Autodesk Inventor part; units mm, degrees
ref_plane "YZ Plane" through (0, 0, 0) normal (1, 0, 0) x (0, 1, 0)
ref_plane "XZ Plane" through (0, 0, 0) normal (0, 1, 0) x (-1, 0, 0)
ref_plane "XY Plane" through (0, 0, 0) normal (0, 0, 1) x (1, 0, 0)
sketch "Sketch1" plane through (0, 0, 0) normal (0, 1, 0) x (-1, 0, 0)
  line L0 (-3, -9) -> (3, -9)
  line L1 (3, -9) -> (3, 9)
  line L2 (3, 9) -> (-3, 9)
  line L3 (-3, 9) -> (-3, -9)
  line L4 (-3, -9) -> (3, 9) construction
  line L5 (3, -9) -> (-3, 9) construction
  circle A0 centre (0, -9) radius 3
  circle A1 centre (0, 9) radius 3
  point P0 (0, 0)
  dimension "d0" = 6
  dimension "d1" = 18
  dimension "d2" = 6
extrude "Extrusion1" add sketch "Sketch1" along normal blind 1.5
sketch "Sketch2" plane through (0, 1.5, 0) normal (0, 1, 0) x (1, 0, 0)
  arc A0 (-3, -9) -> (3, -9) centre (0, -9) ccw
  arc A1 (3, 9) -> (-3, 9) centre (0, 9) ccw
  circle A2 centre (0, 9) radius 1.5
  circle A3 centre (0, -9) radius 1.5
  point P0 (0, 0)
  dimension "d5" = 3
  dimension "d6" = 3
extrude "Extrusion2" cut sketch "Sketch2" against normal blind 2
properties part number "ruka_tahlo"
The listing builds one solid part. Answer for the finished solid, in the listing's coordinates (mm). Round coordinates to 2 decimals unless told otherwise and drop trailing zeros. Order: outer loops, then holes, each group sorted by start corner. A loop starts at its lowest first (then second) coordinate and runs counter-clockwise, first axis right, second up. Notation, with made-up numbers: (17, 77.25) -> (74, 77.25) arc R29 cw to (74, 97.25) -> close; hole circle Ø7 at (76.25, -11). An arc over 180 degrees is marked (long way). Answer as CSV lines item,"result". Start each with the question number.
(1) The part is cut by section C-C (z = 10). Determine the outline of the cut face in (x, y), then the cut area to 3 significant figures.
(2) Find the intervals of material crossed by probe 1 along Z at (x, y) = (0, 0.6); probe 2 along X at (y, z) = (0.9, -9); probe 3 along Z at (x, y) = (-0.4, 0.25), in increasing order. Write a range as from..to.
(3) The part is cut by section B-B (x = 0). Determine the outline of the cut face in (y, z).
(4) For a pull along X with two mould halves and no side action, classify faces 1 (the face through (0, 1, -12)), 2 (the face through (-0.325, 0.76, -7.536)), 3 (the face through (-0.325, 0.76, 10.464)), 4 (the face through (0, 0, 0)) as +X half, -X half, draft (parallel to the pull), parting line (faces both ways), or undercut.
(5) The part is cut by section A-A (y = 0.75). Determine the outline of the cut face in (x, z), then the cut area to 3 significant figures.
(6) The part is cut by section D-D (x = 2.3). Determine the outline of the cut face in (y, z).
Evaluation:
1,outline,"(-2.83, 0) -> (-1.12, 0) -> (-1.12, 1.5) -> (-2.83, 1.5) -> close; (1.12, 0) -> (2.83, 0) -> (2.83, 1.5) -> (1.12, 1.5) -> close"
1,area,"5.13 mm²"
2,probe 1,"-12..-10.5, -7.5..7.5, 10.5..12"
2,probe 2,"-3..-1.5, 1.5..3"
2,probe 3,"-11.97..-10.45, -7.55..7.55, 10.45..11.97"
3,outline,"(0, -12) -> (1.5, -12) -> (1.5, -10.5) -> (0, -10.5) -> close; (0, -7.5) -> (1.5, -7.5) -> (1.5, 7.5) -> (0, 7.5) -> close; (0, 10.5) -> (1.5, 10.5) -> (1.5, 12) -> (0, 12) -> close"
4,face 1,"parting line"
4,face 2,"undercut"
4,face 3,"undercut"
4,face 4,"draft"
5,outline,"(-3, -9) arc R3 ccw to (3, -9) -> (3, 9) arc R3 ccw to (-3, 9) -> close; hole circle Ø3 at (0, -9); hole circle Ø3 at (0, 9)"
5,area,"122 mm²"
6,outline,"(0, -10.93) -> (1.5, -10.93) -> (1.5, 10.93) -> (0, 10.93) -> close"
